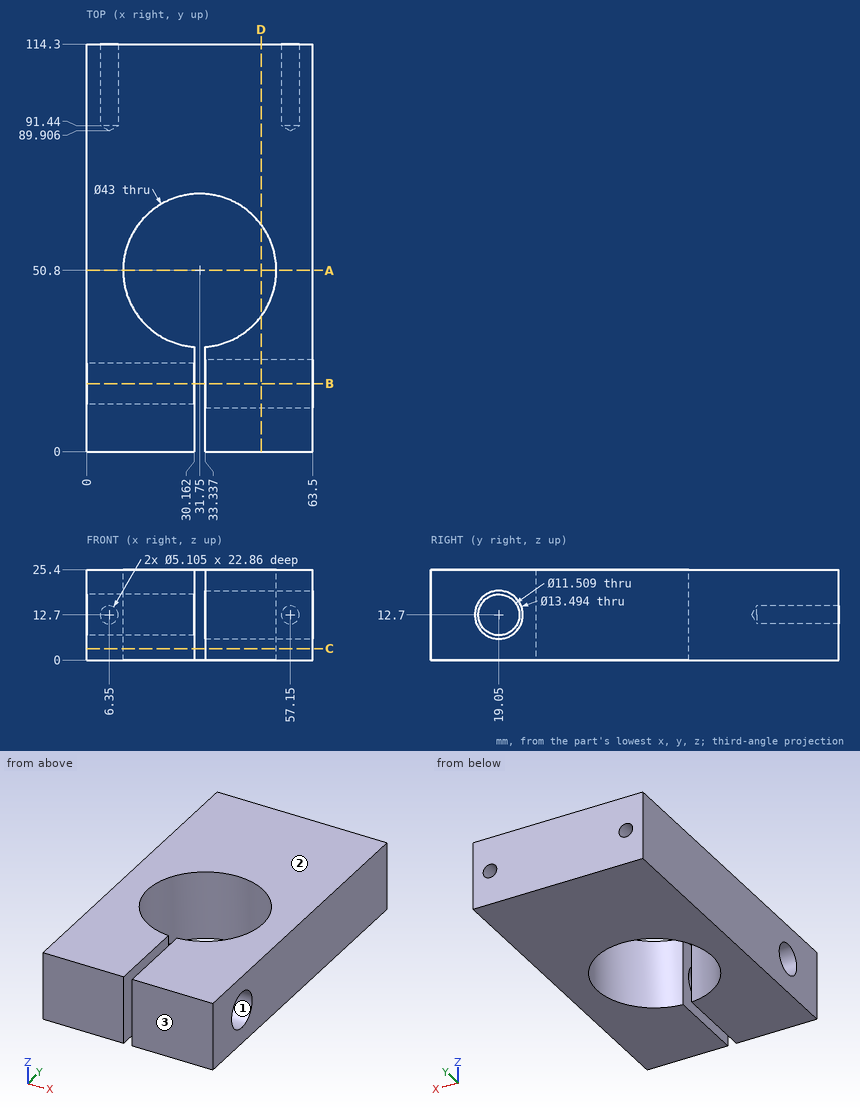
Geometry check sheet. Reference: drawing and pictorial views, mm from the part's lowest x, y, z. Give positions to 0.01 mm unless a question says otherwise; leave off trailing zeros. Loops run counter-clockwise (first coordinate to the right, second up) from the corner with the lowest first, then second, coordinate; pieces in that order, holes last. Notation, with made-up numbers: M 55.25,74.5 L 112.25,74.5 A23 cw 112.25,104.5 Z; hole C 53.5,-23 d6. An arc over 180 degrees is marked long. Use a Markdown table: item, result. Add a question column.
Q1. Sectioned sample at D-D, the plane x = 49. Record the cut outline in (y, z), then the cut area to 3 significant figures.
Q2. Sectioned sample at A-A, the plane y = 50.8. Record the cut outline in (x, z).
Q3. Scan lines: line 1 along X through (y, z) = (108.5, 12.7); line 2 along Z through (x, y) = (16, 19) (1 decimal); line 3 along Z through (x, y) = (55.5, 19.05). Record each from-to range of solid material in increasing order. Write a range as [from, to].
Q4. Sectioned sample at C-C, the plane z = 3.25. Record the cut outline in (x, y), then the cut area to 3 significant figures.
Q5. Go/stop test with flat-tipped pins: pin 1 (3 mm diameter, centred on x = 6.35, z = 12.7, fed in from +Y); pin 2 (10.5 mm diameter, centred on y = 19.05, z = 12.7, fed in from +X). Record where each tip stops, or that it passes through.
Q6. Mould release check, pull along Y, two halves, no side actions. Record for the marked faces 1, 2 and 3: pulls with the +Y half, pulls with the -Y half, needs draft (parallel to the pull), parting line crosses it, or undercut.
Q7. Sectioned sample at B-B, the plane y = 19.05. Record the cut outline in (x, z) (1 decimal).
Verdict:
| question | item | result |
|---|---|---|
| 1 | outline | M 0,0 L 37.97,0 L 37.97,25.4 L 0,25.4 Z; M 63.63,0 L 114.3,0 L 114.3,25.4 L 63.63,25.4 Z; hole C 19.05,12.7 d13.49 |
| 1 | area | 2,110 mm^2 |
| 2 | outline | M 0,0 L 10.25,0 L 10.25,25.4 L 0,25.4 Z; M 53.25,0 L 63.5,0 L 63.5,25.4 L 53.25,25.4 Z |
| 3 | line 1 | [0, 3.8], [8.9, 54.6], [59.7, 63.5] |
| 3 | line 2 | [0, 6.9], [18.5, 25.4] |
| 3 | line 3 | [0, 5.95], [19.45, 25.4] |
| 4 | outline | M 0,0 L 30.16,0 L 30.16,29.36 A21.5 cw long 33.34,29.36 L 33.34,0 L 63.5,0 L 63.5,114.3 L 0,114.3 Z |
| 4 | area | 5,710 mm^2 |
| 5 | pin 1 | y = 90.81 |
| 5 | pin 2 | through |
| 6 | face 1 | undercut |
| 6 | face 2 | needs draft |
| 6 | face 3 | pulls with the -Y half |
| 7 | outline | M 0,0 L 30.2,0 L 30.2,6.9 L 0,6.9 Z; M 0,18.5 L 30.2,18.5 L 30.2,25.4 L 0,25.4 Z; M 33.3,0 L 63.5,0 L 63.5,6 L 33.3,6 Z; M 33.3,19.4 L 63.5,19.4 L 63.5,25.4 L 33.3,25.4 Z |
